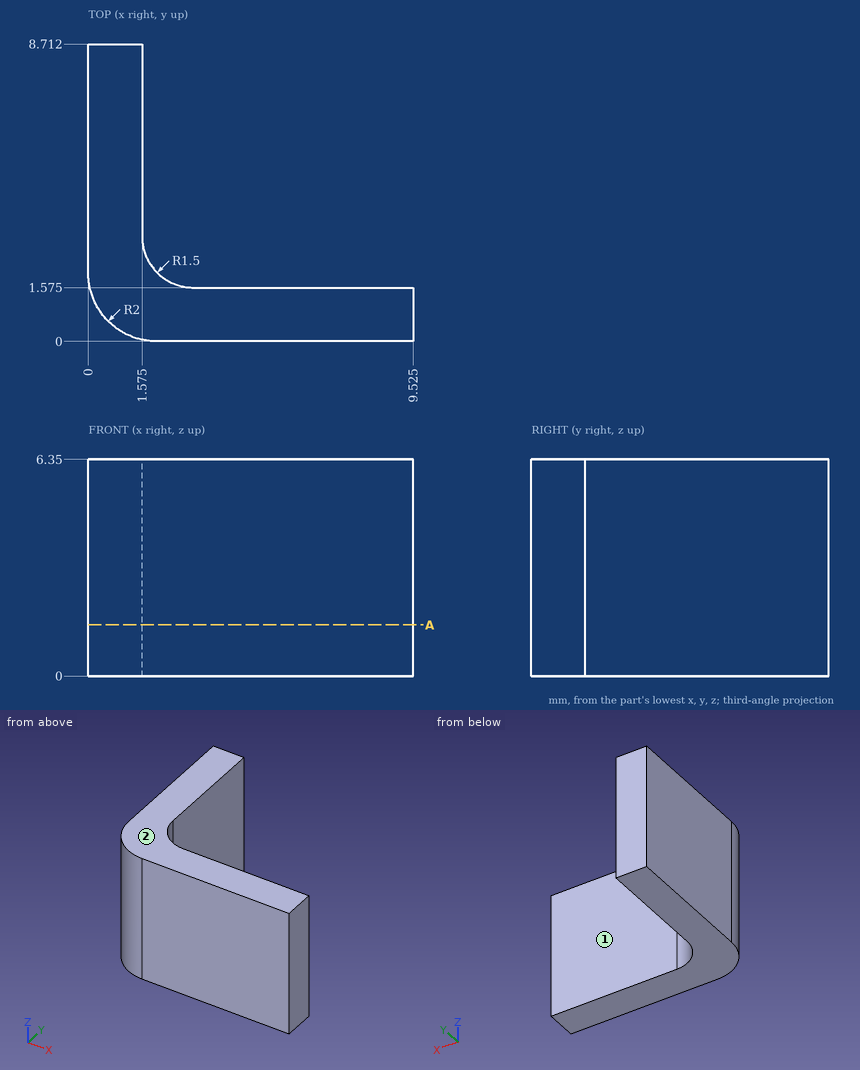
Geometry check sheet. Reference: drawing and pictorial views, mm from the part's lowest x, y, z. A direction names the side the tool comes from. Coordinates: 2 decimals unless noted, no trailing zeros. Order: outer loops, then holes, each group sorted by start corner. A loop starts at its lowest first (then second) coordinate and runs counter-clockwise, first axis right, second up.
Item 1: Depth check by flat-ended pin: pin 1 (2 mm diameter, centred on x = 2.5, z = 3.5, fed in from -Y); pin 2 (1 mm diameter, centred on x = 6.5, z = 1, fed in from +Y) (3 decimals). Enter the tip coordinate at first touch or a pass-through.
Item 2: Tool access check on the marked faces 1 and 2. Record the directions out of +Z, -Z, +X, -X, +Y, -Y that give a thin tool (end or side, any length) a straight path to the whole face; none if there is none.
Item 3: Scan lines: line 1 along Y through (x, z) = (7.75, 2.5) (1 decimal); line 2 along X through (y, z) = (1, 5.25) (1 decimal). Record each from-to range of solid material in increasing order.
Item 4: Section check A-A (z = 1.5). Enter the section's corners in (x, y) (1 decimal), plus the area to 3 significant figures.
Check sheet entries:
1. pin 1: stops at y = 0
1. pin 2: stops at y = 1.575
2. face 1: +Z, -Z, +X, +Y
2. face 2: +Z, +X, -X, +Y, -Y
3. line 1: y = 0 to 1.6
3. line 2: x = 0.3 to 9.5
4. outline: (0, 2) arc R2 ccw to (2, 0) - (9.5, 0) - (9.5, 1.6) - (3.1, 1.6) arc R1.5 cw to (1.6, 3.1) - (1.6, 8.7) - (0, 8.7) - close
4. area: 25.9 mm2
